Source: CAD feature listing. Evaluate the final solid. Frame: model axes, mm. Round coordinates to 2 decimals unless told otherwise and drop trailing zeros. Order: outer loops, then holes, each group sorted by start corner. A loop starts at its lowest first (then second) coordinate and runs counter-clockwise, first axis right, second up. Notation, with made-up numbers: (9.25, 2) -> (44.25, 2) arc R20 cw to (44.25, 31) -> close; hole circle Ø9 at (-26.5, 3.25). An arc over 180 degrees is marked (long way). Use a Markdown table: item, result. Add a question column.
```python
from build123d import *

# Parameters (mm, degrees)
BOSS_EXTRUDE1_DEPTH = 6.35
SKETCH4_W           = 38.1
SKETCH4_H           = 101.6
CUT_EXTRUDE3_DEPTH  = 252.527339468
SKETCH5_W           = 12.7
SKETCH5_H           = 25.4
CUT_EXTRUDE4_DEPTH  = 252.527339468
SKETCH6_W           = 6.35
SKETCH6_H           = 50.8
CUT_EXTRUDE5_DEPTH  = 252.527339468
SKETCH13_W          = 12.7
SKETCH13_H          = 152.4
CUT_EXTRUDE8_DEPTH  = 252.527339468


with BuildPart() as part:
    # Sketch1 → Boss-Extrude1 (new body)
    with BuildSketch(Plane(origin=(0, 0, 0), x_dir=(1, 0, 0), z_dir=(0, 1, 0))):
        Polygon((-177.8, -177.8), (-76.2, -177.8), (-76.2, -168.275), (76.2, -168.275), (76.2, -177.8), (177.8, -177.8), (177.8, -103.124), (168.275, -103.124), (168.275, 49.276), (177.8, 49.276), (177.8, 123.952), (-177.8, 123.952), (-177.8, 49.276), (-168.275, 49.276), (-168.275, -103.124), (-177.8, -103.124), align=None)
    extrude(amount=BOSS_EXTRUDE1_DEPTH)

    # Sketch4 → Cut-Extrude3 (cut, through all)
    with BuildSketch(Plane(origin=(0, 6.35, 0), x_dir=(1, 0, 0), z_dir=(0, 1, 0))):
        with Locations((139.7, -82.423)):
            Rectangle(SKETCH4_W, SKETCH4_H)
        with Locations((-139.7, -82.423)):
            Rectangle(SKETCH4_W, SKETCH4_H)
    extrude(amount=-CUT_EXTRUDE3_DEPTH, mode=Mode.SUBTRACT)

    # Sketch5 → Cut-Extrude4 (cut, through all)
    with BuildSketch(Plane(origin=(0, 6.35, 0), x_dir=(1, 0, 0), z_dir=(0, 1, 0))):
        with Locations((114.3, -120.523)):
            Rectangle(SKETCH5_W, SKETCH5_H)
        with Locations((114.3, -44.323)):
            Rectangle(SKETCH5_W, SKETCH5_H)
        with Locations((-114.3, -44.323)):
            Rectangle(SKETCH5_W, SKETCH5_H)
        with Locations((-114.3, -120.523)):
            Rectangle(SKETCH5_W, SKETCH5_H)
    extrude(amount=-CUT_EXTRUDE4_DEPTH, mode=Mode.SUBTRACT)

    # Sketch6 → Cut-Extrude5 (cut, through all)
    with BuildSketch(Plane(origin=(0, 6.35, 0), x_dir=(1, 0, 0), z_dir=(0, 1, 0))):
        with Locations((117.475, -82.423)):
            Rectangle(SKETCH6_W, SKETCH6_H)
        with Locations((-117.475, -82.423)):
            Rectangle(SKETCH6_W, SKETCH6_H)
    extrude(amount=-CUT_EXTRUDE5_DEPTH, mode=Mode.SUBTRACT)

    # Sketch13 → Cut-Extrude8 (cut, through all)
    with BuildSketch(Plane(origin=(0, 6.35, 0), x_dir=(1, 0, 0), z_dir=(0, 1, 0))):
        with Locations((-28.575, -26.924)):
            Rectangle(SKETCH13_W, SKETCH13_H)
        with Locations((28.575, -26.924)):
            Rectangle(SKETCH13_W, SKETCH13_H)
    extrude(amount=-CUT_EXTRUDE8_DEPTH, mode=Mode.SUBTRACT)


solid = part.part
```
1) Line query: probe 1 along X at (y, z) = (0.75, 91) (3 decimals); probe 2 along X at (y, z) = (3.25, -47) (3 decimals); probe 3 along X at (y, z) = (6.25, 112). Output: solid intervals per line, ascending. Write a range as from..to.
2) Section B-B on z = 89.5. Output: boundary loops of the cut face in (x, y) (3 decimals), then the cut area to 3 significant figures.
3) First-contact query: pin 1 Ø3 at (y, z) = (4, -2.5) entering from +X (3 decimals); pin 2 Ø1.9 at (y, z) = (2.5, 8.5) entering from -X (3 decimals); pin 3 Ø1.9 at (x, y) = (-30, 4.5) entering from +Z (3 decimals). Flat tips, straight axial feed; report the tip coordinate or a pass-through.
4) Section A-A on z = 20. Output: boundary loops of the cut face in (x, y) (3 decimals), then the cut area to 3 significant figures.
5) Section D-D on x = 48. Output: boundary loops of the cut face in (y, z) (3 decimals).
6) Section C-C on y = 1.25. Count the separate pieces of the cut face and the enclosed holes in it, then the cut area to 3 significant figures.
Conclusion:
| question | item | result |
|---|---|---|
| 1 | probe 1 | x = -168.275..-158.75, -114.3..-34.925, -22.225..22.225, 34.925..114.3, 158.75..168.275 |
| 1 | probe 2 | x = -168.275..-34.925, -22.225..22.225, 34.925..168.275 |
| 1 | probe 3 | x = -177.8..-158.75, -107.95..107.95, 158.75..177.8 |
| 2 | outline | (-168.275, 0) -> (-158.75, 0) -> (-158.75, 6.35) -> (-168.275, 6.35) -> close; (-114.3, 0) -> (-34.925, 0) -> (-34.925, 6.35) -> (-114.3, 6.35) -> close; (-22.225, 0) -> (22.225, 0) -> (22.225, 6.35) -> (-22.225, 6.35) -> close; (34.925, 0) -> (114.3, 0) -> (114.3, 6.35) -> (34.925, 6.35) -> close; (158.75, 0) -> (168.275, 0) -> (168.275, 6.35) -> (158.75, 6.35) -> close |
| 2 | area | 1,410 mm^2 |
| 3 | pin 1 | stops at x = 168.275 |
| 3 | pin 2 | stops at x = -168.275 |
| 3 | pin 3 | stops at z = 168.275 |
| 4 | outline | (-168.275, 0) -> (-34.925, 0) -> (-34.925, 6.35) -> (-168.275, 6.35) -> close; (-22.225, 0) -> (22.225, 0) -> (22.225, 6.35) -> (-22.225, 6.35) -> close; (34.925, 0) -> (168.275, 0) -> (168.275, 6.35) -> (34.925, 6.35) -> close |
| 4 | area | 1,980 mm^2 |
| 5 | outline | (0, -123.952) -> (6.35, -123.952) -> (6.35, 168.275) -> (0, 168.275) -> close |
| 6 | separate pieces | 1 |
| 6 | enclosed holes | 4 |
| 6 | area | 89,400 mm^2 |
